Source: CAD feature listing. Evaluate the final solid. Frame: model axes, mm. Face numbers are marked on the shaded views. Round coordinates to 2 decimals unless told otherwise and drop trailing zeros. Write each loop counter-clockwise with the first axis right and the second up, starting at its lowest first coordinate (ties: lowest second). Pieces come first, ordered by that corner, then holes. Notation, with made-up numbers: M 54,55.25 L 79,55.25 A21 cw 79,92.25 Z; hole C 26.25,74.25 d8. An arc over 180 degrees is marked long. Answer in a Markdown table with one row per item. Add a question column.
Item 1: Cut plane A-A on y = -19. Return loops of the section in (x, z).
Item 2: Cut plane C-C on z = 4. Return loops of the section in (x, y).
Item 3: Contact query for flat-ended pins moving along their axis: pin 1 (8 mm diameter, centred on x = -32.79, y = 0, fed in from +Z); pin 2 (1.5 mm diameter, centred on y = -18.5, z = 1.5, fed in from +X); pin 3 (1 mm diameter, centred on x = -19.5, z = 4, fed in from +Y); pin 4 (1.5 mm diameter, centred on y = 2.5, z = 4, fed in from +X). Output: stop coordinate, or through.
Item 4: Cut plane D-D on y = 0. Return loops of the section in (x, z).
Item 5: Mould query, pull axis Y, two halves, no side actions, for the marked faces 1, 2, 3 and 4. Classes: released by +Y, released by -Y, zero draft, split by the parting line, or undercut.
Item 6: Cut plane B-B on x = -26. Return loops of the section in (y, z), and give its area (3 significant figures).
Item 7: Material intervals for probe 1 along Y at (x, z) = (-24, 3.35); probe 2 along Y at (x, z) = (-29, 0.35); probe 3 along X at (y, z) = (0.5, 1.55), sorted ascending.
from build123d import *

# Parameters (mm, degrees)
F0_R     = 13.705866293
F0_R_2   = 4.3874864706
F0_R_3   = 4.303486485
F0_R_4   = 4.6919029461
F0_R_5   = 4.4212893062
F1_DEPTH = 5


# Not quite as in the source:
# - a feature names something its author has since deleted; it is built from what else it names


with BuildPart() as f1:
    # F0 (on Top) → F1 (new body)
    with BuildSketch(Plane.XY):
        with BuildLine():
            ThreePointArc((-21.5933528567, 15.5303339684), (-34.0411472206, -28.1567693277), (7.2290643581, -9.1757204846))
            ThreePointArc((7.2290643581, -9.1757204846), (1.8714254099, 6.2896489682), (-11.9051478269, 15.1263891627))
            ThreePointArc((-11.9051478269, 15.1263891627), (-13.4691027147, 15.4513831507), (-15.0506199283, 15.6758364569))
            ThreePointArc((-15.0506199283, 15.6758364569), (-17.255118812, 13.6982838706), (-19.3682330997, 15.77320015))
            ThreePointArc((-19.3682330997, 15.77320015), (-20.4835124203, 15.6766823614), (-21.5933528567, 15.5303339684))
        make_face()
        with Locations((-17.4914449453, -16.3063649088)):
            Circle(F0_R, mode=Mode.SUBTRACT)
        with Locations((-32.7908843756, 0)):
            Circle(F0_R_2, mode=Mode.SUBTRACT)
        with Locations((-23.3562290668, 6.6427942365)):
            Circle(F0_R_3, mode=Mode.SUBTRACT)
        with Locations((-2.1920050494, 0)):
            Circle(F0_R_4, mode=Mode.SUBTRACT)
        with Locations((-10.8616864309, 6.6427942365)):
            Circle(F0_R_5, mode=Mode.SUBTRACT)
        with BuildLine():
            ThreePointArc((-15.0506199283, 15.6758364569), (-13.4691027147, 15.4513831507), (-11.9051478269, 15.1263891627))
            ThreePointArc((-11.9051478269, 15.1263891627), (-16.560489471, 19.8555989303), (-21.5933528567, 15.5303339684))
            ThreePointArc((-21.5933528567, 15.5303339684), (-20.4835124203, 15.6766823614), (-19.3682330997, 15.77320015))
            ThreePointArc((-19.3682330997, 15.77320015), (-17.2504619715, 18.0246709507), (-15.0426456956, 15.8614274114))
            ThreePointArc((-15.0426456956, 15.8614274114), (-15.044640173, 15.768546317), (-15.0506199283, 15.6758364569))
        make_face()
    extrude(amount=F1_DEPTH)


solid = f1.part
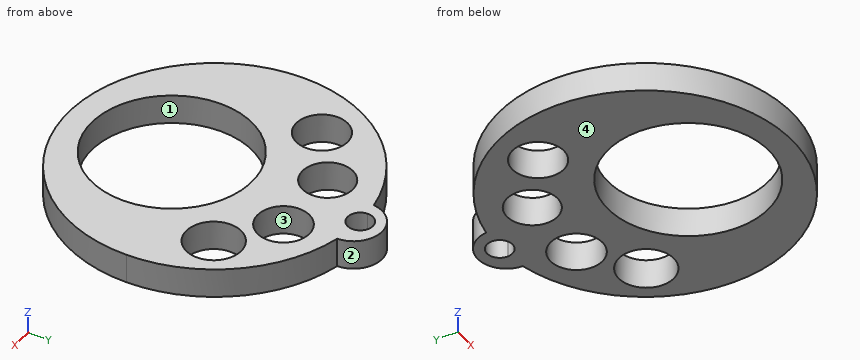
Results below:
| question | item | result |
|---|---|---|
| 1 | outline | M -40.76,0 L -30.93,0 L -30.93,5 L -40.76,5 Z; M -4.05,0 L 5.22,0 L 5.22,5 L -4.05,5 Z |
| 2 | outline | M -21.59,15.53 A25 ccw long -11.91,15.13 A4.86 ccw Z; hole C -32.79,0 d8.77; hole C -17.49,-16.31 d27.41; hole C -23.36,6.64 d8.61; hole C -17.21,15.86 d4.33; hole C -10.86,6.64 d8.84; hole C -2.19,0 d9.38 |
| 3 | pin 1 | through |
| 3 | pin 2 | x = 5.71 |
| 3 | pin 3 | y = 19.31 |
| 3 | pin 4 | x = 4.72 |
| 4 | outline | M -41.03,0 L -37.18,0 L -37.18,5 L -41.03,5 Z; M -28.4,0 L -6.88,0 L -6.88,5 L -28.4,5 Z; M 2.5,0 L 5.48,0 L 5.48,5 L 2.5,5 Z |
| 5 | face 1 | undercut |
| 5 | face 2 | released by +Y |
| 5 | face 3 | undercut |
| 5 | face 4 | zero draft |
| 6 | outline | M -32.78,0 L -27.05,0 L -27.05,5 L -32.78,5 Z; M -5.56,0 L 3.25,0 L 3.25,5 L -5.56,5 Z; M 10.04,0 L 14.43,0 L 14.43,5 L 10.04,5 Z |
| 6 | area | 94.7 mm2 |
| 7 | probe 1 | -33.39 to -28.37, -4.24 to 2.39, 10.9 to 15.04 |
| 7 | probe 2 | -31.51 to -23.75, -8.86 to -2.21, 2.21 to 13.16 |
| 7 | probe 3 | -40.82 to -37.15, -28.43 to -6.86, 2.47 to 5.28 |
